```python
from build123d import *

# Parameters (mm, degrees)
SKIZZE1_R                       = 6.5
AUFSATZ_LINEAR_AUSTRAGEN1_DEPTH = 20
SKIZZE4_R                       = 15
SCHNITT_LINEAR_AUSTRAGEN2_DEPTH = 14.4
M4_GEWINDEBOHRUNG1_D            = 3.3
M4_GEWINDEBOHRUNG1_DEPTH        = 11.5
M4_GEWINDEBOHRUNG1_CSINK_D      = 4.05
M4_GEWINDEBOHRUNG1_CSINK_ANGLE  = 90
M4_GEWINDEBOHRUNG1_TIP          = 0.991420021
SKIZZE7_R                       = 2.25
SCHNITT_LINEAR_AUSTRAGEN3_DEPTH = 20
SKIZZE8_R                       = 4.5
SCHNITT_LINEAR_AUSTRAGEN4_DEPTH = 10
FASE1_SIZE                      = 0.5
FASE2_SIZE                      = 0.5
SKIZZE9_R                       = 1.6
SCHNITT_LINEAR_AUSTRAGEN5_DEPTH = 15
M4_GEWINDEBOHRUNG2_D            = 3.3
M4_GEWINDEBOHRUNG2_DEPTH        = 11.5
M4_GEWINDEBOHRUNG2_CSINK_D      = 4.05
M4_GEWINDEBOHRUNG2_CSINK_ANGLE  = 90
M4_GEWINDEBOHRUNG2_TIP          = 0.991420021
SKIZZE11_R                      = 2.25
SCHNITT_LINEAR_AUSTRAGEN6_DEPTH = 30
SKIZZE12_R                      = 4.5
SCHNITT_LINEAR_AUSTRAGEN7_DEPTH = 10
FASE3_SIZE                      = 0.5


with BuildPart() as part:
    # Skizze1 → Aufsatz-Linear austragen1 (new body)
    with BuildSketch(Plane.XY):
        with BuildLine():
            Line((0, 0), (100, 0))
            Line((100, 0), (77.53225634, 51.915320425))
            ThreePointArc((77.53225634, 51.915320425), (50, 70), (22.46774366, 51.915320425))
            Line((22.46774366, 51.915320425), (0, 0))
        make_face()
        with Locations((50, 40)):
            Circle(SKIZZE1_R, mode=Mode.SUBTRACT)
    extrude(amount=AUFSATZ_LINEAR_AUSTRAGEN1_DEPTH)

    # Skizze4 → Schnitt-Linear austragen2 (cut)
    with BuildSketch(Plane(origin=(0, 0, 0), x_dir=(-1, 0, 0), z_dir=(0, 0, -1))):
        with Locations((-50, 40)):
            Circle(SKIZZE4_R)
    extrude(amount=-SCHNITT_LINEAR_AUSTRAGEN2_DEPTH, mode=Mode.SUBTRACT)

    # M4 Gewindebohrung1
    with Locations(Plane(origin=(38.375, 5.29, 20), x_dir=(1, 0, 0), z_dir=(0, 0, 1))):
        with Locations((0, 0), (23.25, 0)):
            CounterSinkHole(M4_GEWINDEBOHRUNG1_D / 2, M4_GEWINDEBOHRUNG1_CSINK_D / 2, depth=M4_GEWINDEBOHRUNG1_DEPTH, counter_sink_angle=M4_GEWINDEBOHRUNG1_CSINK_ANGLE)
            with Locations((0, 0, -(M4_GEWINDEBOHRUNG1_DEPTH + M4_GEWINDEBOHRUNG1_TIP / 2))):  # 118° drill point
                Cone(0, M4_GEWINDEBOHRUNG1_D / 2, M4_GEWINDEBOHRUNG1_TIP, mode=Mode.SUBTRACT)

    # Skizze7 → Schnitt-Linear austragen3 (cut)
    with BuildSketch(Plane(origin=(0, 0, 0), x_dir=(-1, 0, 0), z_dir=(0, 0, -1))):
        with Locations((-30.48202317, 32)):
            Circle(SKIZZE7_R)
        with Locations((-30.48202317, 14)):
            Circle(SKIZZE7_R)
    extrude(amount=-SCHNITT_LINEAR_AUSTRAGEN3_DEPTH, mode=Mode.SUBTRACT)

    # Skizze8 → Schnitt-Linear austragen4 (cut)
    with BuildSketch(Plane.XY.offset(20)):
        with Locations((30.48202317, 32)):
            Circle(SKIZZE8_R)
        with Locations((30.48202317, 14)):
            Circle(SKIZZE8_R)
    extrude(amount=-SCHNITT_LINEAR_AUSTRAGEN4_DEPTH, mode=Mode.SUBTRACT)

    # Fase1
    fase1_edges = [part.edges().sort_by_distance(p)[0] for p in [
        (43.5, 40, 20),
        (25.98202317, 32, 20),
        (25.98202317, 14, 20),
    ]]
    chamfer(fase1_edges, length=FASE1_SIZE)

    # Fase2
    fase2_edges = [part.edges().sort_by_distance(p)[0] for p in [
        (65, 40, 0),
        (32.73202317, 32, 0),
        (32.73202317, 14, 0),
    ]]
    chamfer(fase2_edges, length=FASE2_SIZE)

    # Skizze9 → Schnitt-Linear austragen5 (cut)
    with BuildSketch(Plane(origin=(0, 0, 0), x_dir=(-1, 0, 0), z_dir=(0, 0, -1))):
        with Locations((-50, 60)):
            Circle(SKIZZE9_R)
        with Locations((-70, 40)):
            Circle(SKIZZE9_R)
        with Locations((-50, 20)):
            Circle(SKIZZE9_R)
    extrude(amount=-SCHNITT_LINEAR_AUSTRAGEN5_DEPTH, mode=Mode.SUBTRACT)

    # M4 Gewindebohrung2
    with Locations(Plane(origin=(70, 40, 0), x_dir=(-1, 0, 0), z_dir=(0, 0, -1))):
        with Locations((0, 0), (20, 20), (20, -20)):
            CounterSinkHole(M4_GEWINDEBOHRUNG2_D / 2, M4_GEWINDEBOHRUNG2_CSINK_D / 2, depth=M4_GEWINDEBOHRUNG2_DEPTH, counter_sink_angle=M4_GEWINDEBOHRUNG2_CSINK_ANGLE)
            with Locations((0, 0, -(M4_GEWINDEBOHRUNG2_DEPTH + M4_GEWINDEBOHRUNG2_TIP / 2))):  # 118° drill point
                Cone(0, M4_GEWINDEBOHRUNG2_D / 2, M4_GEWINDEBOHRUNG2_TIP, mode=Mode.SUBTRACT)

    # Skizze11 → Schnitt-Linear austragen6 (cut)
    with BuildSketch(Plane(origin=(0, 0, 0), x_dir=(-1, 0, 0), z_dir=(0, 0, -1))):
        with Locations((-80.50404106, 29)):
            Circle(SKIZZE11_R)
        with Locations((-80.50404106, 17)):
            Circle(SKIZZE11_R)
    extrude(amount=-SCHNITT_LINEAR_AUSTRAGEN6_DEPTH, mode=Mode.SUBTRACT)

    # Skizze12 → Schnitt-Linear austragen7 (cut)
    with BuildSketch(Plane.XY.offset(20)):
        with Locations((80.50404106, 29)):
            Circle(SKIZZE12_R)
        with Locations((80.50404106, 17)):
            Circle(SKIZZE12_R)
    extrude(amount=-SCHNITT_LINEAR_AUSTRAGEN7_DEPTH, mode=Mode.SUBTRACT)

    # Fase3
    fase3_edges = [part.edges().sort_by_distance(p)[0] for p in [
        (76.00404106, 29, 20),
        (76.00404106, 17, 20),
    ]]
    chamfer(fase3_edges, length=FASE3_SIZE)


solid = part.part
```
Work out the finished part from the listing and answer in its coordinate system (mm). A direction names the side the tool comes from. Round coordinates to 2 decimals unless told otherwise and drop trailing zeros. Write each loop counter-clockwise with the first axis right and the second up, starting at its lowest first coordinate (ties: lowest second). Pieces come first, ordered by that corner, then holes. Notation, with made-up numbers: (17.5, 78) - (54.5, 78) arc R26 cw to (54.5, 98) - close; hole circle Ø3 at (-24, 24). An arc over 180 degrees is marked (long way). Return JSON: item names as keys, results as strings. Group by question number.
Q1. The part is cut by section B-B on z = 2.5. Count the separate pieces of the cut face and the enclosed holes in it, then the cut area to 3 significant figures.
Q2. The part is cut by section C-C on y = 40. Write down the section's boundary in (x, z) (3 decimals).
Q3. For faces 4 (the cylindrical face through (49.14, 21.35, 13.24)), 5 (the cylindrical face through (63.273, 5.363, 13.985)), 6 (the flat face through (11.39, 26.32, 9.86)), determine the directions among +Z, -Z, +X, -X, +Y, -Y from which every point of the face is accessible in a straight line to the end or side of a thin tool.
Q4. Find the intervals of material crossed by L1, parallel to X at y = 30, z = 7.25; L2, parallel to X at y = 19.5, z = 12; L3, parallel to X at y = 40, z = 19.25, in increasing order.
Q5. The mould has two halves that part along X. Classify faces 1 (the flat face through (49, 28, 20)), 2 (the conical face through (38.09, 5.3, 7.68)), 3 (the cylindrical face through (50, 70, 10)): released by +X, released by -X, zero draft, split by the parting line, or undercut.
Q6. The part is cut by section A-A on z = 16. Write down the section's boundary in (x, y) (3 decimals), then the cut area to 3 significant figures.
Q7. The part is cut by section D-D on y = 60. Write down the section's boundary in (x, z) (3 decimals).
Q8. Each of these flat-tipped pins is pushed along its axis until it touches: pin 1 Ø10.5 at (x, y) = (30.48, 32) entering from +Z; pin 2 Ø1.5 at (y, z) = (60.5, 8) entering from +X; pin 3 Ø4.5 at (x, y) = (81, 30) entering from +Z; pin 4 Ø8 at (x, y) = (50, 40) entering from -Z. Where does it stop, or does it pass through?
Solved:
{
 "1": {"separate pieces": "1", "enclosed holes": "8", "area": "3,950 mm²"},
 "2": {"outline": "(17.311, 0) - (34.5, 0) - (35, 0.5) - (35, 14.4) - (43.5, 14.4) - (43.5, 19.5) - (43, 20) - (17.311, 20) - close; (56.5, 14.4) - (65, 14.4) - (65, 0.5) - (65.5, 0) - (67.975, 0) - (68.35, 0.375) - (68.35, 11.5) - (68.4, 11.53) - (68.4, 15) - (71.6, 15) - (71.6, 11.53) - (71.65, 11.5) - (71.65, 0.375) - (72.025, 0) - (82.689, 0) - (82.689, 20) - (57, 20) - (56.5, 19.5) - close"},
 "3": {"face 4": "-Z", "face 5": "+Z", "face 6": "+Z, -Z, -X, +Y"},
 "4": {"L1": "12.98 to 29.45, 31.51 to 38.82, 61.18 to 78.49, 82.52 to 87.02", "L2": "8.44 to 48.48, 51.52 to 76.76, 84.25 to 91.56", "L3": "17.31 to 43.5, 56.5 to 82.69"},
 "5": {"face 1": "zero draft", "face 2": "undercut", "face 3": "split by the parting line"},
 "6": {"outline": "(0, 0) - (100, 0) - (77.532, 51.915) arc R30 ccw to (22.468, 51.915) - close; hole circle Ø9 at (30.482, 14); hole circle Ø9 at (30.482, 32); hole circle Ø3.3 at (38.375, 5.29); hole circle Ø13 at (50, 40); hole circle Ø3.3 at (61.625, 5.29); hole circle Ø9 at (80.504, 17); hole circle Ø9 at (80.504, 29)", "area": "4,340 mm²"},
 "7": {"outline": "(27.639, 0) - (47.975, 0) - (48.35, 0.375) - (48.35, 11.5) - (48.4, 11.53) - (48.4, 15) - (51.6, 15) - (51.6, 11.53) - (51.65, 11.5) - (51.65, 0.375) - (52.025, 0) - (72.361, 0) - (72.361, 20) - (27.639, 20) - close"},
 "8": {"pin 1": "z = 20", "pin 2": "x = 72.58", "pin 3": "z = 10", "pin 4": "through"}
}
